from build123d import *

# Parameters (mm, degrees)
SKETCH_1_R          = 27
SKETCH_1_R_2        = 3.175
EXTRUDE_1_DEPTH     = 16
CUT_EXTRUDE_START   = -7.5
SKETCH_2_R          = 27
SKETCH_2_R_2        = 10
CUT_EXTRUDE_1_DEPTH = 7.5
SKETCH_3_R          = 15
CUT_EXTRUDE_2_DEPTH = 6
CUT_EXTRUDE_START_2 = -6
SKETCH_4_R          = 27
SKETCH_4_R_2        = 17.8
CUT_EXTRUDE_3_DEPTH = 6
SKETCH_5_R          = 2
CUT_EXTRUDE_4_DEPTH = 16.25
EXTRUDE_START       = 1.5
SKETCH_6_R          = 27
SKETCH_6_R_2        = 15
EXTRUDE_5_DEPTH     = 1.5
SKETCH_7_R          = 2
CUT_EXTRUDE_6_DEPTH = 41.500000033
CHAMFER_1_SIZE      = 1.5
SKETCH_8_R          = 2
CUT_EXTRUDE_7_DEPTH = 43.002976085


with BuildPart() as part:
    # Эскиз1 → Вытянуть1 (new body)
    with BuildSketch(Plane(origin=(0, 0, 0), x_dir=(1, 0, 0), z_dir=(0, 1, 0))):
        with Locations(Location((0, 0, 0), (0, 0, 270))):
            Circle(SKETCH_1_R)
        with Locations(Location((0, 0, 0), (0, 0, 270))):
            Circle(SKETCH_1_R_2, mode=Mode.SUBTRACT)
    extrude(amount=EXTRUDE_1_DEPTH)

    # Эскиз2 → Вырез-Вытянуть1 (cut)
    with BuildSketch(Plane(origin=(0, 16, 0), x_dir=(1, 0, 0), z_dir=(0, 1, 0)).offset(CUT_EXTRUDE_START)):
        with Locations(Location((0, 0, 0), (0, 0, 270))):
            Circle(SKETCH_2_R)
        with Locations(Location((0, 0, 0), (0, 0, 270))):
            Circle(SKETCH_2_R_2, mode=Mode.SUBTRACT)
    extrude(amount=CUT_EXTRUDE_1_DEPTH, mode=Mode.SUBTRACT)

    # Эскиз3 → Вытянуть2 (cut)
    with BuildSketch(Plane.XZ):
        with Locations(Location((0, 0, 0), (0, 0, 270))):
            Circle(SKETCH_3_R)
    extrude(amount=-CUT_EXTRUDE_2_DEPTH, mode=Mode.SUBTRACT)

    # Эскиз4 → Вытянуть3 (cut)
    with BuildSketch(Plane(origin=(0, 8.5, 0), x_dir=(1, 0, 0), z_dir=(0, 1, 0)).offset(CUT_EXTRUDE_START_2)):
        with Locations(Location((0, 0, 0), (0, 0, 270))):
            Circle(SKETCH_4_R)
        with Locations(Location((0, 0, 0), (0, 0, 270))):
            Circle(SKETCH_4_R_2, mode=Mode.SUBTRACT)
    extrude(amount=CUT_EXTRUDE_3_DEPTH, mode=Mode.SUBTRACT)

    # Эскиз5 → Вытянуть4 (cut, symmetric)
    with BuildSketch(Plane.XY):
        with Locations((0, 11)):
            Circle(SKETCH_5_R)
    extrude(amount=CUT_EXTRUDE_4_DEPTH, both=True, mode=Mode.SUBTRACT)

    # Эскиз6 → Вытянуть5 (add)
    with BuildSketch(Plane.XZ.offset(EXTRUDE_START)):
        with Locations(Location((0, 0, 0), (0, 0, 270))):
            Circle(SKETCH_6_R)
        with Locations(Location((0, 0, 0), (0, 0, 270))):
            Circle(SKETCH_6_R_2, mode=Mode.SUBTRACT)
    extrude(amount=-EXTRUDE_5_DEPTH)

    # Эскиз7 → Вытянуть6 (cut, through all)
    with BuildSketch(Plane(origin=(0, 2.5, 0), x_dir=(1, 0, 0), z_dir=(0, 1, 0))):
        with Locations(Location((0, 22.5, 0), (0, 0, 270))):
            Circle(SKETCH_7_R)
        with Locations(Location((22.5, 0, 0), (0, 0, 270))):
            Circle(SKETCH_7_R)
        with Locations(Location((0, -22.5, 0), (0, 0, 270))):
            Circle(SKETCH_7_R)
        with Locations(Location((-22.5, 0, 0), (0, 0, 270))):
            Circle(SKETCH_7_R)
    extrude(amount=-CUT_EXTRUDE_6_DEPTH, mode=Mode.SUBTRACT)

    # Фаска1
    chamfer_1_edges = [part.edges().sort_by_distance(p)[0] for p in [
        (0, -1.5, -24.5),
        (22.5, -1.5, -2),
        (0, -1.5, 20.5),
        (-22.5, -1.5, -2),
    ]]
    chamfer(chamfer_1_edges, length=CHAMFER_1_SIZE)

    # Эскиз8 → Вытянуть7 (cut, through all)
    with BuildSketch(Plane(origin=(0, 16, 0), x_dir=(1, 0, 0), z_dir=(0, 1, 0))):
        with Locations(Location((-6.60744303, 0, 0), (0, 0, 270))):
            Circle(SKETCH_8_R)
        with Locations(Location((6.60744303, 0, 0), (0, 0, 90))):
            Circle(SKETCH_8_R)
    extrude(amount=-CUT_EXTRUDE_7_DEPTH, mode=Mode.SUBTRACT)


solid = part.part
Design review of the part built by this model. Coordinates are the model's own, in mm. A direction names the side the tool comes from. Round coordinates to 2 decimals unless told otherwise and drop trailing zeros. Write each loop counter-clockwise with the first axis right and the second up, starting at its lowest first coordinate (ties: lowest second). Pieces come first, ordered by that corner, then holes.
Item 1: For faces 5 (the cylindrical face through (-2, 11, -6)), 6 (the flat face through (-18, 2.5, 6)), list the 3-axis set-ups (+Z, -Z, +X, -X, +Y, -Y) from which the entire face can be reached by the end or side of a thin tool; tool diameter is ignored.
Item 2: Consider section B-B on z = -22.5. Give the boundary of the cut face in (x, y), and give its area (3 significant figures).
Item 3: Consider section A-A on y = 11. Give the boundary of the cut face in (x, z) (3 decimals), and give its area (3 significant figures).
Item 4: Consider section C-C on x = -22.5. Give the boundary of the cut face in (y, z).
Item 5: Draft analysis for pull direction Z (two halves, no side actions). For faces 1 (the flat face through (-12, -1.5, -12)), 2 (the cylindrical face through (21.3, 1.3, -1.6)), 3 (the cylindrical face through (3, 12.2, 9.54)), 4 (the cylindrical face through (-1.2, 1.3, -24.1)), state which applies: released by +Z, released by -Z, zero draft, split by the parting line, or undercut.
Item 6: Consider section D-D on y = 1.25. Give the boundary of the cut face in (x, z), and give its area (3 significant figures).
Item 7: For pin 1 Ø1 at (y, z) = (8.5, 10.5) entering from -X; pin 2 Ø5 at (y, z) = (8.5, 4.5) entering from +X; pin 3 Ø3 at (x, z) = (-6.5, 17.5) entering from +Y, all flat-tipped, find the tip position at first contact; note any pin that passes through.
Item 8: Wall thickness on L1, parallel to X at y = 2, z = 0; L2, parallel to X at y = 10.25, z = 0 (3 decimals); L3, parallel to Y at x = 0, z = 6: over which ranges is each line inside the solid? List them lowest first.
Check values:
1. face 5: +Z, -Z
1. face 6: +Y
2. outline: (-14.92, -1.5) - (-3.5, -1.5) - (-2, 0) - (-2, 2.5) - (-14.92, 2.5) - close; (2, 0) - (3.5, -1.5) - (14.92, -1.5) - (14.92, 2.5) - (2, 2.5) - close
2. area: 101 mm2
3. outline: (-2, -9.798) - (-2, -2.466) arc R3.175 cw to (-2, 2.466) - (-2, 9.798) arc R10 ccw to start; (2, -9.798) arc R10 ccw to (2, 9.798) - (2, 2.466) arc R3.175 cw to (2, -2.466) - close; hole circle Ø4 at (-6.607, 0); hole circle Ø4 at (6.607, 0)
3. area: 201 mm2
4. outline: (-1.5, -14.92) - (2.5, -14.92) - (2.5, -2) - (0, -2) - (-1.5, -3.5) - close; (-1.5, 3.5) - (0, 2) - (2.5, 2) - (2.5, 14.92) - (-1.5, 14.92) - close
5. face 1: zero draft
5. face 2: undercut
5. face 3: split by the parting line
5. face 4: undercut
6. outline: circle Ø54 at (0, 0); hole circle Ø4 at (-22.5, 0); hole circle Ø30 at (0, 0); hole circle Ø4 at (0, -22.5); hole circle Ø4 at (0, 22.5); hole circle Ø4 at (22.5, 0)
6. area: 1,530 mm2
7. pin 1: stops at x = -14.73
7. pin 2: stops at x = 17.69
7. pin 3: stops at y = 8.5
8. L1: x = -27 to -24.5, -20.5 to -15, 15 to 20.5, 24.5 to 27
8. L2: x = -10 to -8.607, -4.607 to -3.175, 3.175 to 4.607, 8.607 to 10
8. L3: y = 6 to 9, 13 to 16
